from build123d import *

# Parameters (mm, degrees)
SKETCH1_R           = 11.5
SKETCH1_R_2         = 4.5
BOSS_EXTRUDE1_DEPTH = 5
BOSS_EXTRUDE2_DEPTH = 12
BOSS_EXTRUDE3_DEPTH = 15


with BuildPart() as part:
    # Sketch1 → Boss-Extrude1 (new body)
    # profile 1 of 3: a face of its own
    with BuildSketch(Plane.XY):
        with BuildLine():
            ThreePointArc((25.426510923, 65.374052201), (25.278878582, 66.375106712), (25.187732235, 67.382875429))
            Line((25.187732235, 67.382875429), (24.689110868, 66.519237886))
            ThreePointArc((24.689110868, 66.519237886), (21.653079074, 64.189608755), (17.858983849, 64.689110868))
            Line((17.858983849, 64.689110868), (-16.782032303, 84.689110868))
            ThreePointArc((-16.782032303, 84.689110868), (-17.613984793, 85.291223321), (-18.305370958, 86.05061092))
            Line((-18.305370958, 86.05061092), (-20.487509935, 82.271035343))
            ThreePointArc((-20.487509935, 82.271035343), (-22.844860879, 77.215679929), (-24.28854511, 71.827777028))
            Line((-24.28854511, 71.827777028), (-36.010847543, 5.347296355))
            ThreePointArc((-36.010847543, 5.347296355), (-35.573320923, 3.714424781), (-34.041232037, 3))
            Line((-34.041232037, 3), (34.041232037, 3))
            ThreePointArc((34.041232037, 3), (35.573320923, 3.714424781), (36.010847543, 5.347296355))
            Line((36.010847543, 5.347296355), (25.426510923, 65.374052201))
        make_face()
        with Locations((0, 20)):
            Circle(SKETCH1_R, mode=Mode.SUBTRACT)
        with Locations((0, 45)):
            Circle(SKETCH1_R_2, mode=Mode.SUBTRACT)
    # profile 2 of 3: a face of its own
    with BuildSketch(Plane.XY):
        with BuildLine():
            ThreePointArc((-38.965270802, 5.868240888), (-37.871454253, 1.786061952), (-34.041232037, 0))
            Line((-34.041232037, 0), (34.041232037, 0))
            ThreePointArc((34.041232037, 0), (37.871454253, 1.786061952), (38.965270802, 5.868240888))
            Line((38.965270802, 5.868240888), (28.380934182, 65.894996734))
            ThreePointArc((28.380934182, 65.894996734), (28.380934182, 71.104442064), (30.162669421, 75.999719399))
            Line((30.162669421, 75.999719399), (25.187732235, 67.382875429))
            ThreePointArc((25.187732235, 67.382875429), (25.278878582, 66.375106712), (25.426510923, 65.374052201))
            Line((25.426510923, 65.374052201), (36.010847543, 5.347296355))
            ThreePointArc((36.010847543, 5.347296355), (35.573320923, 3.714424781), (34.041232037, 3))
            Line((34.041232037, 3), (-34.041232037, 3))
            ThreePointArc((-34.041232037, 3), (-35.573320923, 3.714424781), (-36.010847543, 5.347296355))
            Line((-36.010847543, 5.347296355), (-24.28854511, 71.827777028))
            ThreePointArc((-24.28854511, 71.827777028), (-22.844860879, 77.215679929), (-20.487509935, 82.271035343))
            Line((-20.487509935, 82.271035343), (-18.305370958, 86.05061092))
            ThreePointArc((-18.305370958, 86.05061092), (-19.274182883, 88.739179708), (-18.612159322, 91.519237886))
            Line((-18.612159322, 91.519237886), (-23.085586146, 83.771035343))
            ThreePointArc((-23.085586146, 83.771035343), (-25.663938741, 78.241740359), (-27.242968369, 72.348721561))
            Line((-27.242968369, 72.348721561), (-38.965270802, 5.868240888))
        make_face()
    # profile 3 of 3: a face of its own
    with BuildSketch(Plane.XY):
        with BuildLine():
            ThreePointArc((-16.782032303, 84.689110868), (-19.111661434, 87.725142661), (-18.612159322, 91.519237886))
            Line((-18.612159322, 91.519237886), (-3.612159322, 117.5))
            Line((-3.612159322, 117.5), (5.048094716, 112.5))
            Line((5.048094716, 112.5), (-7.451905284, 90.849364905))
            Line((-7.451905284, 90.849364905), (18.52885683, 75.849364905))
            Line((18.52885683, 75.849364905), (31.02885683, 97.5))
            Line((31.02885683, 97.5), (39.689110868, 92.5))
            Line((39.689110868, 92.5), (30.162669421, 75.999719399))
            Line((30.162669421, 75.999719399), (24.689110868, 66.519237886))
            ThreePointArc((24.689110868, 66.519237886), (21.653079074, 64.189608755), (17.858983849, 64.689110868))
            Line((17.858983849, 64.689110868), (-16.782032303, 84.689110868))
        make_face()
    extrude(amount=BOSS_EXTRUDE1_DEPTH)

    # Sketch1_3 → Boss-Extrude2 (add)
    with BuildSketch(Plane.XY):
        with BuildLine():
            ThreePointArc((-38.965270802, 5.868240888), (-37.871454253, 1.786061952), (-34.041232037, 0))
            Line((-34.041232037, 0), (34.041232037, 0))
            ThreePointArc((34.041232037, 0), (37.871454253, 1.786061952), (38.965270802, 5.868240888))
            Line((38.965270802, 5.868240888), (28.380934182, 65.894996734))
            ThreePointArc((28.380934182, 65.894996734), (28.380934182, 71.104442064), (30.162669421, 75.999719399))
            Line((30.162669421, 75.999719399), (25.187732235, 67.382875429))
            ThreePointArc((25.187732235, 67.382875429), (25.278878582, 66.375106712), (25.426510923, 65.374052201))
            Line((25.426510923, 65.374052201), (36.010847543, 5.347296355))
            ThreePointArc((36.010847543, 5.347296355), (35.573320923, 3.714424781), (34.041232037, 3))
            Line((34.041232037, 3), (-34.041232037, 3))
            ThreePointArc((-34.041232037, 3), (-35.573320923, 3.714424781), (-36.010847543, 5.347296355))
            Line((-36.010847543, 5.347296355), (-24.28854511, 71.827777028))
            ThreePointArc((-24.28854511, 71.827777028), (-22.844860879, 77.215679929), (-20.487509935, 82.271035343))
            Line((-20.487509935, 82.271035343), (-18.305370958, 86.05061092))
            ThreePointArc((-18.305370958, 86.05061092), (-19.274182883, 88.739179708), (-18.612159322, 91.519237886))
            Line((-18.612159322, 91.519237886), (-23.085586146, 83.771035343))
            ThreePointArc((-23.085586146, 83.771035343), (-25.663938741, 78.241740359), (-27.242968369, 72.348721561))
            Line((-27.242968369, 72.348721561), (-38.965270802, 5.868240888))
        make_face()
    extrude(amount=BOSS_EXTRUDE2_DEPTH)

    # Sketch1_4 → Boss-Extrude3 (add)
    with BuildSketch(Plane.XY):
        with BuildLine():
            ThreePointArc((-16.782032303, 84.689110868), (-19.111661434, 87.725142661), (-18.612159322, 91.519237886))
            Line((-18.612159322, 91.519237886), (-3.612159322, 117.5))
            Line((-3.612159322, 117.5), (5.048094716, 112.5))
            Line((5.048094716, 112.5), (-7.451905284, 90.849364905))
            Line((-7.451905284, 90.849364905), (18.52885683, 75.849364905))
            Line((18.52885683, 75.849364905), (31.02885683, 97.5))
            Line((31.02885683, 97.5), (39.689110868, 92.5))
            Line((39.689110868, 92.5), (30.162669421, 75.999719399))
            Line((30.162669421, 75.999719399), (24.689110868, 66.519237886))
            ThreePointArc((24.689110868, 66.519237886), (21.653079074, 64.189608755), (17.858983849, 64.689110868))
            Line((17.858983849, 64.689110868), (-16.782032303, 84.689110868))
        make_face()
    extrude(amount=BOSS_EXTRUDE3_DEPTH)


solid = part.part
Verification items for the finished model (mm, model axes). A direction names the side the tool comes from. Round coordinates to 2 decimals unless told otherwise and drop trailing zeros. Loops run counter-clockwise (first coordinate to the right, second up) from the corner with the lowest first, then second, coordinate; pieces in that order, holes last. Notation, with made-up numbers: (70.5, 49) - (105.5, 49) arc R30 ccw to (105.5, 83) - close; hole circle Ø7 at (-16.75, 39.5). An arc over 180 degrees is marked (long way). Answer in a Markdown table with one row per item. Add a question column.
Q1. Tool access check on faces 4 (the face through (-30.232, 38.122, 8.451)), 5 (the face through (5.357, 83.454, 7.395)), 6 (the face through (24.69, 86.52, 7.4)). Record the directions out of +Z, -Z, +X, -X, +Y, -Y that give a thin tool (end or side, any length) a straight path to the whole face; none if there is none.
Q2. Release check for a two-part mould opening along X. For faces 1 (the face through (21.706, 64.204, 9.93)), 2 (the face through (37.8, 1.7, 5.9)), 3 (the face through (0, 0, 6)) record: pulls with the +X half, pulls with the -X half, needs draft (parallel to the pull), parting line crosses it, or undercut.
Q3. Section check C-C on y = 45. Enter the section's corners in (x, z), plus the area to 3 significant figures.
Q4. Section check D-D on y = 20. Enter the section's corners in (x, z).
Q5. Material ranges on line 1 (Y direction, x = 0, z = 2.65); line 2 (X direction, y = 85.5, z = 9.5); line 3 (Z direction, x = -4, y = 72), recorded low to high.
Q6. Gauge pin test, flat ends, axial feed: pin 1 (8 mm diameter, centred on y = 75, z = 6, fed in from +X); pin 2 (6 mm diameter, centred on x = 12.5, y = 37.5, fed in from +Z); pin 3 (2 mm diameter, centred on x = 6, z = 8.5, fed in from +Y); pin 4 (5 mm diameter, centred on x = 22.5, y = 56.5, fed in from -Z). Record the tip position at first contact, or that the pin passes through.
Q7. Section check A-A on z = 10.75. Enter the section's corners in (x, y) (1 decimal).
Q8. Section check B-B on x = 0. Enter the section's corners in (y, z).
Found:
| question | item | result |
|---|---|---|
| 1 | face 4 | +Z |
| 1 | face 5 | +Z, -Z |
| 1 | face 6 | +Z, -Z, +Y |
| 2 | face 1 | undercut |
| 2 | face 2 | pulls with the +X half |
| 2 | face 3 | needs draft |
| 3 | outline | (-32.07, 0) - (-4.5, 0) - (-4.5, 5) - (-29.02, 5) - (-29.02, 12) - (-32.07, 12) - close; (4.5, 0) - (32.07, 0) - (32.07, 12) - (29.02, 12) - (29.02, 5) - (4.5, 5) - close |
| 3 | area | 318 mm² |
| 4 | outline | (-36.47, 0) - (-11.5, 0) - (-11.5, 5) - (-33.43, 5) - (-33.43, 12) - (-36.47, 12) - close; (11.5, 0) - (36.47, 0) - (36.47, 12) - (33.43, 12) - (33.43, 5) - (11.5, 5) - close |
| 5 | line 1 | y = 0 to 8.5, 31.5 to 40.5, 49.5 to 86.55, 103.76 to 115.41 |
| 5 | line 2 | x = -22.09 to -18.62, -17.83 to 1.81, 24.1 to 35.65 |
| 5 | line 3 | z = 0 to 5 |
| 6 | pin 1 | stops at x = 31.89 |
| 6 | pin 2 | stops at z = 5 |
| 6 | pin 3 | stops at y = 112.53 |
| 6 | pin 4 | stops at z = 0 |
| 7 | outline | (-39, 5.9) arc R5 ccw to (-34, 0) - (34, 0) arc R5 ccw to (39, 5.9) - (28.4, 65.9) arc R15 cw to (30.2, 76) - (39.7, 92.5) - (31, 97.5) - (18.5, 75.8) - (-7.5, 90.8) - (5, 112.5) - (-3.6, 117.5) - (-23.1, 83.8) arc R35 ccw to (-27.2, 72.3) - close; hole (-36, 5.3) arc R2 ccw to (-34, 3) - (34, 3) arc R2 ccw to (36, 5.3) - (25.4, 65.4) arc R18 cw to (25.2, 67.4) - (24.7, 66.5) arc R5 cw to (17.9, 64.7) - (-16.8, 84.7) arc R5 cw to (-18.3, 86.1) - (-20.5, 82.3) arc R32 ccw to (-24.3, 71.8) - close |
| 8 | outline | (0, 0) - (8.5, 0) - (8.5, 5) - (3, 5) - (3, 12) - (0, 12) - close; (31.5, 0) - (40.5, 0) - (40.5, 5) - (31.5, 5) - close; (49.5, 0) - (86.55, 0) - (86.55, 15) - (75, 15) - (75, 5) - (49.5, 5) - close; (103.76, 0) - (115.41, 0) - (115.41, 15) - (103.76, 15) - close |
